```python
from build123d import *

# Parameters (mm, degrees)
F0_W     = 38.1
F0_H     = 57.15
F1_DEPTH = 41.402
F2_R     = 2.794
F3_DEPTH = 38.101
F4_R     = 1.984375
F5_DEPTH = 25.4
F6_W     = 12.7
F6_H     = 4.064
F7_DEPTH = 15.748
F8_R     = 4.468898
F8_R_2   = 4.064
F9_DEPTH = 32.767


with BuildPart() as f1:
    # F0 (on Top) → F1 (new body)
    with BuildSketch(Plane.XY):
        with Locations((19.05, 28.575)):
            Rectangle(F0_W, F0_H)
    extrude(amount=F1_DEPTH)

    # F2 (on face) → F3 (cut, through all)
    with BuildSketch(Plane.YZ.offset(38.1)):
        with Locations((14.732, 14.732)):
            Circle(F2_R)
        with Locations((42.418, 14.732)):
            Circle(F2_R)
    extrude(amount=-F3_DEPTH, mode=Mode.SUBTRACT)

    # F4 (on face) → F5 (cut)
    with BuildSketch(Plane.XY.offset(41.402)):
        with Locations((19.05, 28.575)):
            Circle(F4_R)
    extrude(amount=-F5_DEPTH, mode=Mode.SUBTRACT)

    # F6 (on face) → F7 (join)
    with BuildSketch(Plane(origin=(0, 0, 0), x_dir=(0, -1, 0), z_dir=(-1, 0, 0))):
        with Locations((-44.45, 30.734)):
            Rectangle(F6_W, F6_H)
        with Locations((-12.7, 30.734)):
            Rectangle(F6_W, F6_H)
    extrude(amount=F7_DEPTH)

    # F8 (on face) → F9 (cut, through all)
    with BuildSketch(Plane.XY.offset(32.766)):
        with Locations((-9.398, 44.45)):
            Circle(F8_R)
        with Locations((-9.398, 12.7)):
            Circle(F8_R_2)
    extrude(amount=-F9_DEPTH, mode=Mode.SUBTRACT)


solid = f1.part
```
Model file for the job. Use its own axes, mm. A direction names the side the tool comes from. Coordinates: 2 decimals unless noted, no trailing zeros. Loops run counter-clockwise (first coordinate to the right, second up) from the corner with the lowest first, then second, coordinate; pieces in that order, holes last. Notation, with made-up numbers: M 70.5,87.25 L 91.5,87.25 A18 ccw 91.5,94.25 Z; hole C 75,61 d2. An arc over 180 degrees is marked long. Use CSV: the item, a comma, the result in double quotes. Start each with the question number.
1. Two-plate mould, pull along Z, no slides. Class faces 1 (the cylindrical face through (19.32, 40.2, 13.03)), 2 (the flat face through (-15.748, 45, 31)), 3 (the flat face through (19, 29, 16.002)), 4 (the flat face through (-4, 45, 28.702)): pulls with the +Z half, pulls with the -Z half, needs draft (parallel to the pull), parting line crosses it, or undercut.
2. Band-saw the part on C-C, the plane x = 24.5. List the corners of the cut face in (y, z).
3. Band-saw the part on D-D, the plane z = 34. List the corners of the cut face in (x, y) (3 decimals).
4. Tool access for faces 5 (the cylindrical face through (18.62, 26.638, 28.88)), 6 (the flat face through (-4, 45, 32.766)), 7 (the flat face through (-8, 6.35, 31)), 8 (the flat face through (-8, 38.1, 31)), 9 (the flat face through (-8, 50.8, 31)): list every direction of +Z, -Z, +X, -X, +Y, -Y with a clear straight run to the whole face (end or side of a thin tool).
5. Flat gauge pins, fed straight in: pin 1 (14 mm diameter, centred on x = -9.5, y = 11, fed in from -Z); pin 2 (3.5 mm diameter, centred on x = 19.05, y = 28.575, fed in from +Z); pin 3 (3.5 mm diameter, centred on x = -5, z = 31, fed in from -Y). Where does each tip first touch, or does it go through?
6. Band-saw the part on A-A, the plane y = 44.45. List the corners of the cut face in (x, z).
7. Band-saw the part on B-B, the plane x = -11.5. List the corners of the cut face in (y, z), then the cut area to 3 significant figures.
8. Probe probe 1 along Y at (x, z) = (17, 15); probe 2 along Y at (x, z) = (19.05, 25.25); probe 3 along X at (y, z) = (35.5, 12.5). List the from-to ranges inside material, lowest first. Write a range as [from, to].
Entries:
1,face 1,"undercut"
1,face 2,"needs draft"
1,face 3,"pulls with the +Z half"
1,face 4,"pulls with the -Z half"
2,outline,"M 0,0 L 57.15,0 L 57.15,41.4 L 0,41.4 Z; hole C 14.73,14.73 d5.59; hole C 42.42,14.73 d5.59"
3,outline,"M 0,0 L 38.1,0 L 38.1,57.15 L 0,57.15 Z; hole C 19.05,28.575 d3.969"
4,face 5,"+Z"
4,face 6,"+Z, -X, +Y, -Y"
4,face 7,"+Z, -Z, -X, -Y"
4,face 8,"+Z, -Z, -X"
4,face 9,"+Z, -Z, -X, +Y"
5,pin 1,"stops at z = 28.7"
5,pin 2,"stops at z = 16"
5,pin 3,"stops at y = 6.35"
6,outline,"M -15.75,28.7 L -13.87,28.7 L -13.87,32.77 L -15.75,32.77 Z; M -4.93,28.7 L 0,28.7 L 0,16.65 L 38.1,16.65 L 38.1,41.4 L 0,41.4 L 0,32.77 L -4.93,32.77 Z; M 0,0 L 38.1,0 L 38.1,12.81 L 0,12.81 Z"
7,outline,"M 6.35,28.7 L 9.22,28.7 L 9.22,32.77 L 6.35,32.77 Z; M 16.18,28.7 L 19.05,28.7 L 19.05,32.77 L 16.18,32.77 Z; M 38.1,28.7 L 40.51,28.7 L 40.51,32.77 L 38.1,32.77 Z; M 48.39,28.7 L 50.8,28.7 L 50.8,32.77 L 48.39,32.77 Z"
7,area,"42.9 mm2"
8,probe 1,"y = [0, 11.95], [17.51, 39.64], [45.2, 57.15]"
8,probe 2,"y = [0, 26.59], [30.56, 57.15]"
8,probe 3,"x = [0, 38.1]"
